Study the drawing (mm; zero at the part's minimum x, y, z) and answer. Round coordinates to 2 decimals unless told otherwise and drop trailing zeros. Order: outer loops, then holes, each group sorted by start corner. A loop starts at its lowest first (then second) coordinate and runs counter-clockwise, first axis right, second up. Notation, with made-up numbers: M 6.25,67 L 57.25,67 A14 cw 57.25,92 Z; hole C 12,5.5 d9. An arc over 180 degrees is marked long. Put each result on its own line as item: value. Start each with the question number.
1. The part is cut by section C-C (x = 9). Give the vertices of the cut face in (y, z).
2. The part is cut by section B-B (y = 4.5). Give the vertices of the cut face in (x, z), then the cut area to 3 significant figures.
3. The part is cut by section A-A (z = 1.05). Give the vertices of the cut face in (x, y), then the cut area to 3 significant figures.
4. Each of these flat-tipped pins is pushed along its axis until it touches: pin 1 Ø0.5 at (y, z) = (1.5, 1) entering from -X; pin 2 Ø0.8 at (y, z) = (1.5, 2.5) entering from +X. Where does it stop, or does it pass through?
5. The mould has two halves that part along X. Classify the marked faces 1, 2 and 3: +X half, -X half, draft (parallel to the pull), parting line (faces both ways), or undercut.
6. The part is cut by section D-D (y = 1.5). Give the vertices of the cut face in (x, z).
7. Consider line 1 (X direction, y = 4.25, z = 0.65); line 2 (X direction, y = 4.5, z = 0.45); line 3 (Y direction, x = 9, z = 3.3). Determine where each line is inside the solid, lowest interval first.
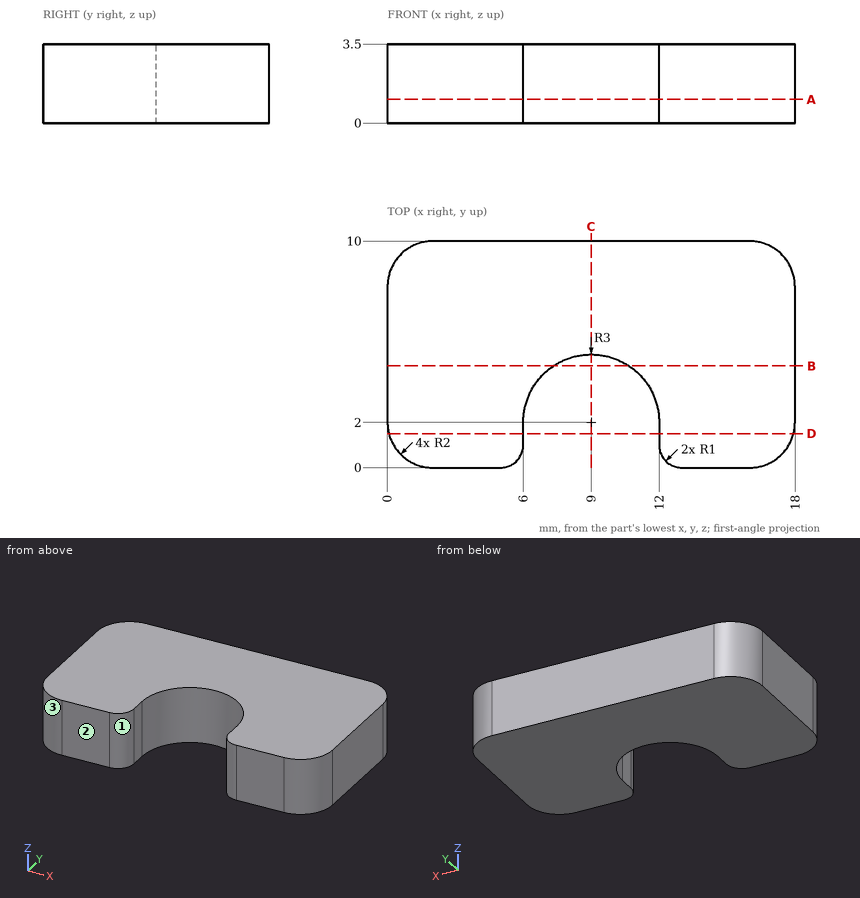
Resolved:
1. outline: M 5,0 L 10,0 L 10,3.5 L 5,3.5 Z
2. outline: M 0,0 L 7.34,0 L 7.34,3.5 L 0,3.5 Z; M 10.66,0 L 18,0 L 18,3.5 L 10.66,3.5 Z
2. area: 51.4 mm2
3. outline: M 0,2 A2 ccw 2,0 L 5,0 A1 ccw 6,1 L 6,2 A3 cw 12,2 L 12,1 A1 ccw 13,0 L 16,0 A2 ccw 18,2 L 18,8 A2 ccw 16,10 L 2,10 A2 ccw 0,8 Z
3. area: 150 mm2
4. pin 1: x = 0.02
4. pin 2: x = 18
5. face 1: undercut
5. face 2: draft
5. face 3: -X half
6. outline: M 0.06,0 L 6,0 L 6,3.5 L 0.06,3.5 Z; M 12,0 L 17.94,0 L 17.94,3.5 L 12,3.5 Z
7. line 1: 0 to 7.02, 10.98 to 18
7. line 2: 0 to 7.34, 10.66 to 18
7. line 3: 5 to 10
